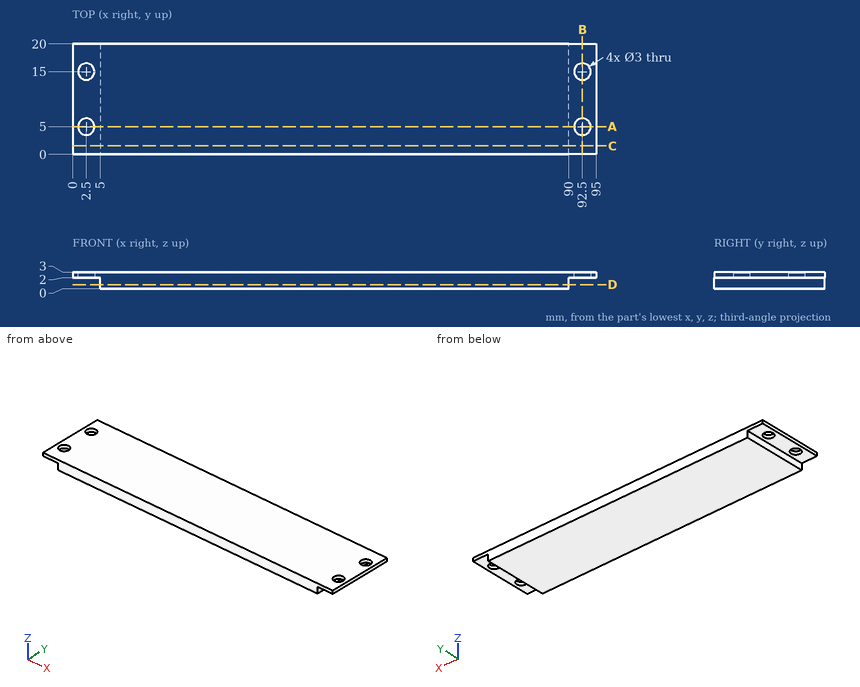
The figure shows three views and two pictorial views of one solid part (mm, origin at its lowest corner). Answer the questions. Round coordinates to 2 decimals unless told otherwise and drop trailing zeros. Write each loop counter-clockwise with the first axis right and the second up, starting at its lowest first coordinate (ties: lowest second). Pieces come first, ordered by that corner, then holes. Notation, with made-up numbers: M 23.25,59 L 75.25,59 A8 ccw 75.25,68 Z; hole C 5.25,-30 d2. An arc over 180 degrees is marked long. Use a Markdown table: item, result.
1) Straight lines are drawn through the part: line 1 along Y through (x, z) = (92.5, 2.6); line 2 along X through (y, z) = (17.5, 0.7). For each, find the intervals that lie inside material, in ascending order. Write a range as [from, to].
Answers follow:
| item | result |
|---|---|
| line 1 | y = [0, 3.5], [6.5, 13.5], [16.5, 20] |
| line 2 | x = [5, 90] |
2) The part is cut by section D-D (z = 0.75). Write down the section's boundary in (x, y), plus the area to 3 significant figures.
Answers follow:
| item | result |
|---|---|
| outline | M 5,0 L 90,0 L 90,20 L 5,20 Z |
| area | 1,700 mm2 |
3) The part is cut by section B-B (x = 92.5). Write down the section's boundary in (y, z), plus the area to 3 significant figures.
Answers follow:
| item | result |
|---|---|
| outline | M 0,2 L 3.5,2 L 3.5,3 L 0,3 Z; M 6.5,2 L 13.5,2 L 13.5,3 L 6.5,3 Z; M 16.5,2 L 20,2 L 20,3 L 16.5,3 Z |
| area | 14.0 mm2 |
4) The part is cut by section C-C (y = 1.5). Write down the section's boundary in (x, z), plus the area to 3 significant figures.
Answers follow:
| item | result |
|---|---|
| outline | M 0,2 L 5,2 L 5,0 L 90,0 L 90,2 L 95,2 L 95,3 L 0,3 Z |
| area | 265 mm2 |
5) Flat-ended cylindrical pins translate along their axes: pin 1 (0.6 mm diameter, centred on y = 13, z = 1, fed in from -X); pin 2 (0.6 mm diameter, centred on y = 10.5, z = 0.5, fed in from +X); pin 3 (4 mm diameter, centred on x = 93, y = 12.5, fed in from -Z). Find the tip coordinate at first contact, or state that the pin passes through.
Answers follow:
| item | result |
|---|---|
| pin 1 | stops at x = 5 |
| pin 2 | stops at x = 90 |
| pin 3 | stops at z = 2 |
6) The part is cut by section A-A (y = 5). Write down the section's boundary in (x, z), plus the area to 3 significant figures.
Answers follow:
| item | result |
|---|---|
| outline | M 0,2 L 1,2 L 1,3 L 0,3 Z; M 4,2 L 5,2 L 5,0 L 90,0 L 90,2 L 91,2 L 91,3 L 4,3 Z; M 94,2 L 95,2 L 95,3 L 94,3 Z |
| area | 259 mm2 |
